Design review of the part built by this model. Coordinates are the model's own, in mm. Coordinates: 2 decimals unless noted, no trailing zeros. Write each loop counter-clockwise with the first axis right and the second up, starting at its lowest first coordinate (ties: lowest second). Pieces come first, ordered by that corner, then holes.
Q1. Add section A-A, the plane z = 0. Give the boundary of the cut face in (x, y).
Q2. The part is to be moulded in two halves that separate along Z. For faces 1 (the face through (88.9, -3, 50)), 2 (the face through (-1, -3, 127)), 3 (the face through (-1, -3, -25.4)), 4 (the face through (-11.34, -3.13, 33.27)), say which applies: +Z half, -Z half, draft (parallel to the pull), parting line (faces both ways), or undercut.
Q3. Add section C-C, the plane y = -4.75. Give the number of separate pieces and of enclosed holes in the cut face, plus the area to 3 significant figures.
Q4. To check wall thickness, follow probe 1 along X at (y, z) = (-2, 54.5); probe 2 along X at (y, z) = (-3.25, 56.5); probe 3 along X at (y, z) = (-3.5, 60). State the ranges of each line that lie inside material, in increasing order.
Q5. Clearance check with a flat-ended pin moving along its axis: pin 1 Ø5 at (x, z) = (51, 3.5) entering from +Y. State where the tip first meets the part, or that it passes through.
Q6. Add section B-B, the plane x = -56.5. Give the boundary of the cut face in (y, z).
from build123d import *

# Parameters (mm, degrees)
F0_W     = 177.8
F0_H     = 101.6
F0_R     = 14.2875
F0_H_2   = 50.8
F1_DEPTH = 6.35


with BuildPart() as f1:
    # F0 (on Front) → F1 (new body)
    with BuildSketch(Plane.XZ):
        with Locations((0, 76.2)):
            Rectangle(F0_W, F0_H)
        with Locations((-62.933081, 50.8)):
            Circle(F0_R, mode=Mode.SUBTRACT)
        with Locations((0, 41.9608)):
            Circle(F0_R, mode=Mode.SUBTRACT)
        with BuildLine():
            ThreePointArc((42.165347, 40.935914), (37.376426, 39.983338), (41.436277, 42.696044))
            ThreePointArc((41.436277, 42.696044), (41.975868, 41.88849), (42.165347, 40.935914))
        make_face(mode=Mode.SUBTRACT)
        with BuildLine():
            ThreePointArc((6.186256, 76.892011), (1.397336, 75.939435), (5.457187, 78.652141))
            ThreePointArc((5.457187, 78.652141), (5.996777, 77.844587), (6.186256, 76.892011))
        make_face(mode=Mode.SUBTRACT)
        with Locations((38.97307, 76.2)):
            Circle(F0_R, mode=Mode.SUBTRACT)
        with BuildLine():
            ThreePointArc((62.126788, 63.386554), (63.503295, 61.326466), (63.98666, 58.896426))
            ThreePointArc((63.98666, 58.896426), (60.066699, 53.029791), (53.146531, 54.406298))
            ThreePointArc((53.146531, 54.406298), (53.146531, 63.386554), (62.126788, 63.386554))
        make_face(mode=Mode.SUBTRACT)
        with BuildLine():
            ThreePointArc((78.086372, 76.856938), (76.549747, 74.557218), (73.837042, 75.096808))
            ThreePointArc((73.837042, 75.096808), (74.644596, 79.156659), (78.086372, 76.856938))
        make_face(mode=Mode.SUBTRACT)
        with BuildLine():
            ThreePointArc((26.147697, 99.342651), (27.524204, 97.282563), (28.007569, 94.852523))
            ThreePointArc((28.007569, 94.852523), (24.087609, 88.985888), (17.167441, 90.362395))
            ThreePointArc((17.167441, 90.362395), (17.167441, 99.342651), (26.147697, 99.342651))
        make_face(mode=Mode.SUBTRACT)
        with BuildLine():
            ThreePointArc((42.107281, 112.813035), (40.570657, 110.513314), (37.857951, 111.052905))
            ThreePointArc((37.857951, 111.052905), (38.665505, 115.112756), (42.107281, 112.813035))
        make_face(mode=Mode.SUBTRACT)
        Rectangle(F0_W, F0_H_2)
        Circle(F0_R, mode=Mode.SUBTRACT)
    extrude(amount=F1_DEPTH)


solid = f1.part
Here are the results:
1. outline: (-88.9, -6.35) - (-14.29, -6.35) - (-14.29, 0) - (-88.9, 0) - close; (14.29, -6.35) - (88.9, -6.35) - (88.9, 0) - (14.29, 0) - close
2. face 1: draft
2. face 2: +Z half
2. face 3: -Z half
2. face 4: undercut
3. separate pieces: 1
3. enclosed holes: 10
3. area: 24,200 mm2
4. probe 1: x = -88.9 to -76.73, -49.13 to -6.85, 6.85 to 53.05, 62.22 to 88.9
4. probe 2: x = -88.9 to -76.03, -49.83 to 51.76, 63.52 to 88.9
4. probe 3: x = -88.9 to -73.86, -52 to 51.38, 63.89 to 88.9
5. pin 1: stops at y = 0
6. outline: (-6.35, -25.4) - (0, -25.4) - (0, 38.04) - (-6.35, 38.04) - close; (-6.35, 63.56) - (0, 63.56) - (0, 127) - (-6.35, 127) - close
